Verification items for the finished model (mm, model axes). A direction names the side the tool comes from. Coordinates: 2 decimals unless noted, no trailing zeros. Order: outer loops, then holes, each group sorted by start corner. A loop starts at its lowest first (then second) coordinate and runs counter-clockwise, first axis right, second up. Notation, with made-up numbers: (78.25, -23.75) -> (124.25, -23.75) arc R15 ccw to (124.25, -14.75) -> close; hole circle Ø6 at (3.5, 22.25). An arc over 180 degrees is marked (long way). Write each question's results on one line, items separated by ' | '. Start each with the question number.
(1) Go/stop test with flat-tipped pins: pin 1 (3 mm diameter, centred on y = 19, z = 3.5, fed in from -X); pin 2 (3 mm diameter, centred on y = 18, z = -1, fed in from +X); pin 3 (12 mm diameter, centred on x = 17, z = -44.5, fed in from +Y). Record where each tip stops, or that it passes through.
(2) Cross-section at C-C on y = 2. Enter the section's corners in (x, z).
(3) Set-up check for faces 1 (the flat face through (36, 20, 29.393)), 2 (the flat face through (36, 20, -31.595)), 3 (the flat face through (6.182, 20, -1)), 4 (the cylindrical face through (92.66, 9.58, -54.96)), 5 (the flat face through (66.548, 20, -1)): record each of +Z, -Z, +X, -X, +Y, -Y from which the full face is reachable in a straight line by a thin tool's end or side.
(4) Cross-section at A-A on z = -11. Enter the section's corners in (x, y), and give its area (3 significant figures).
(5) Cross-section at B-B on x = 24.5. Enter the section's corners in (y, z), and give its area (3 significant figures).
(6) Cross-section at D-D on z = 42. Enter the section's corners in (x, y), and give its area (3 significant figures).
(7) Thickness scan on probe 1 along Y at (x, z) = (24.5, -35.5); probe 2 along X at (y, z) = (15.5, -30.5); probe 3 along Z at (x, y) = (33, 20.5). Record the ranges inside material, lowest first. Write a range as [from, to].
```python
from build123d import *

# Parameters (mm, degrees)
SKETCH2_W           = 115
SKETCH2_H           = 110
BOSS_EXTRUDE1_DEPTH = 15
SKETCH3_W           = 60.365616492
SKETCH3_H           = 60.987942435
BOSS_EXTRUDE2_DEPTH = 10
FILLET2_R           = 4


with BuildPart() as part:
    # Sketch2 → Boss-Extrude1 (new body)
    with BuildSketch(Plane(origin=(0, 0, 0), x_dir=(1, 0, 0), z_dir=(0, 1, 0))):
        with Locations((36.364864865, 1.101351351)):
            Rectangle(SKETCH2_W, SKETCH2_H)
    extrude(amount=BOSS_EXTRUDE1_DEPTH)

    # Sketch3 → Boss-Extrude2 (add)
    with BuildSketch(Plane(origin=(0, 15, 0), x_dir=(1, 0, 0), z_dir=(0, 1, 0))):
        with Locations((36.364864865, 1.101351351)):
            Rectangle(SKETCH3_W, SKETCH3_H)
    extrude(amount=BOSS_EXTRUDE2_DEPTH)

    # Fillet2
    fillet2_edges = [part.edges().sort_by_distance(p)[0] for p in [
        (36.364864865, 0, -56.101351351),
        (93.864864865, 0, -1.101351351),
        (36.364864865, 0, 53.898648649),
        (-21.135135135, 0, -1.101351351),
        (-21.135135135, 7.5, -56.101351351),
        (93.864864865, 7.5, -56.101351351),
        (93.864864865, 7.5, 53.898648649),
        (-21.135135135, 7.5, 53.898648649),
    ]]
    fillet(fillet2_edges, radius=FILLET2_R)


solid = part.part
```
Results are:
1) pin 1: stops at x = 6.18 | pin 2: stops at x = 66.55 | pin 3: stops at y = 15
2) outline: (-20.6, -52.1) arc R3.46 ccw to (-17.14, -55.57) -> (89.86, -55.57) arc R3.46 ccw to (93.33, -52.1) -> (93.33, 49.9) arc R3.46 ccw to (89.86, 53.36) -> (-17.14, 53.36) arc R3.46 ccw to (-20.6, 49.9) -> close
3) face 1: +Z, +X, -X, +Y | face 2: -Z, +X, -X, +Y | face 3: +Z, -Z, -X, +Y | face 4: -Z, +X, +Y, -Y | face 5: +Z, -Z, +X, +Y
4) outline: (-21.14, 4) arc R4 ccw to (-17.14, 0) -> (89.86, 0) arc R4 ccw to (93.86, 4) -> (93.86, 15) -> (66.55, 15) -> (66.55, 25) -> (6.18, 25) -> (6.18, 15) -> (-21.14, 15) -> close | area: 2,320 mm2
5) outline: (0, -52.1) arc R4 ccw to (4, -56.1) -> (15, -56.1) -> (15, -31.6) -> (25, -31.6) -> (25, 29.39) -> (15, 29.39) -> (15, 53.9) -> (4, 53.9) arc R4 ccw to (0, 49.9) -> close | area: 2,250 mm2
6) outline: (-21.14, 4) arc R4 ccw to (-17.14, 0) -> (89.86, 0) arc R4 ccw to (93.86, 4) -> (93.86, 15) -> (-21.14, 15) -> close | area: 1,720 mm2
7) probe 1: y = [0, 15] | probe 2: x = [6.18, 66.55] | probe 3: z = [-31.6, 29.39]
